Autodesk Inventor part; units mm, degrees
ref_plane "YZ Plane" through (0, 0, 0) normal (1, 0, 0) x (0, 1, 0)
ref_plane "XZ Plane" through (0, 0, 0) normal (0, 1, 0) x (-1, 0, 0)
ref_plane "XY Plane" through (0, 0, 0) normal (0, 0, 1) x (1, 0, 0)
sketch "Sketch1" plane through (0, 0, 0) normal (0, 0, 1) x (1, 0, 0)
  line L0 (5.5, 2.5) -> (5.5, 8)
  line L1 (5.5, 8) -> (3.5, 8)
  line L2 (3.5, 8) -> (3.5, 6.07)
  line L3 (3.5, 6.07) -> (0, 6.07)
  line L4 (5.5, 2.5) -> (0, 2.5)
  line L5 (0, 2.5) -> (0, 6.07)
  line L6 (-2.3, 0) -> (6.8, 0)
  line L7 (0, 0) -> (0, 17.5)
  line L8 (0, 9) -> (0, 2.5)
  line L9 (0, 15) -> (0, 9)
  point P0 (0, 4.285)
  point P1 (-1, 12)
  point P2 (4.5, 8)
  dimension "d0" = 5.5
  dimension "d1" = 3.5
  dimension "d2" = 6.07
  dimension "d3" = 8
  dimension "d4" = 2.5
  dimension "d8" = 1
revolve "Revolution1" add sketch "Sketch1" angle 360 about axis through (-10, 0, 0) along (1, 0, 0)
mirror "Mirror2" about plane through (0, 0, 0) normal (1, 0, 0) of "Revolution1"
properties part number "Idler_Pulley" material "Aluminum 6061"
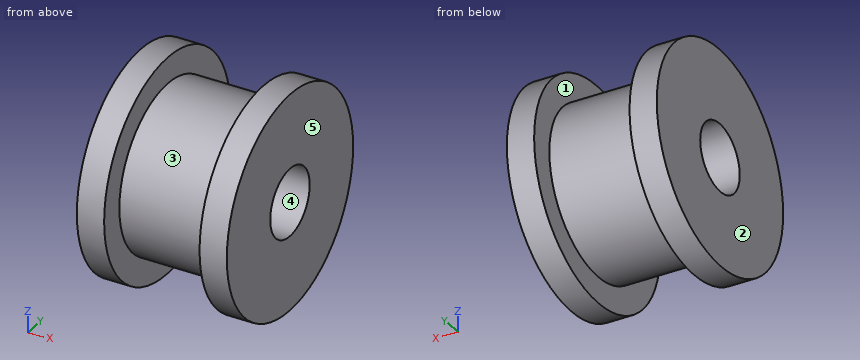
Can you work these out from the model? Positions are in its coordinate system, mm. Face numbers are marked on the shaded views. A direction names the side the tool comes from. Round coordinates to 2 decimals unless told otherwise and drop trailing zeros. Loops run counter-clockwise (first coordinate to the right, second up) from the corner with the lowest first, then second, coordinate; pieces in that order, holes last. Notation, with made-up numbers: (10.5, 49) -> (51.5, 49) arc R18 cw to (51.5, 83) -> close; hole circle Ø10 at (43, -12.75). An arc over 180 degrees is marked (long way). One line per item, written item: value. Start each with the question number.
1. For the marked faces 1 and 2, which set-ups out of +Z, -Z, +X, -X, +Y, -Y let a thin tool reach every point of the face, with its end or its side?
2. If we section it at A-A, the plane z = 0: Write out the boundary of the cut face in (x, y), then the cut area to 3 significant figures.
3. If we mould it in two halves opening along X, with no side actions, what happens to the marked faces 3, 4 and 5? For each: pulls with the +X half, pulls with the -X half, needs draft (parallel to the pull), parting line crosses it, or undercut.
4. If we section it at C-C, the plane x = -1: Write out the boundary of the cut face in (y, z).
5. If I drill on probe 1 along Z at (x, y) = (2.5, 0); probe 2 along X at (y, z) = (-5.75, -3.25); probe 3 along Y at (x, z) = (-3, -2.25), over which ranges is the centre line in solid material (lowest first)?
6. For pin 1 (1.5 mm diameter, centred on x = 2, y = 3.5, fed in from +Z); pin 2 (5 mm diameter, centred on x = -3.5, y = -5, fed in from +Z); pin 3 (2 mm diameter, centred on x = 0, y = -6.5, fed in from -Z); pin 4 (4 mm diameter, centred on y = 0, z = 0, fed in from +X), each with a flat end and sliding along its axis, tell me the tip position at first contact or that it passes through.
7. If we section it at D-D, the plane z = -5: Write out the boundary of the cut face in (x, y) (3 decimals).
Calculated:
1. face 1: none
1. face 2: +Z, -Z, -X, +Y, -Y
2. outline: (-5.5, -8) -> (-3.5, -8) -> (-3.5, -6.07) -> (3.5, -6.07) -> (3.5, -8) -> (5.5, -8) -> (5.5, -2.5) -> (-5.5, -2.5) -> close; (-5.5, 2.5) -> (5.5, 2.5) -> (5.5, 8) -> (3.5, 8) -> (3.5, 6.07) -> (-3.5, 6.07) -> (-3.5, 8) -> (-5.5, 8) -> close
2. area: 94.0 mm²
3. face 3: undercut
3. face 4: needs draft
3. face 5: pulls with the +X half
4. outline: circle Ø12.14 at (0, 0); hole circle Ø5 at (0, 0)
5. probe 1: z = -6.07 to -2.5, 2.5 to 6.07
5. probe 2: x = -5.5 to -3.5, 3.5 to 5.5
5. probe 3: y = -5.64 to -1.09, 1.09 to 5.64
6. pin 1: stops at z = 5.41
6. pin 2: stops at z = 7.6
6. pin 3: stops at z = -2.57
6. pin 4: passes through
7. outline: (-5.5, -6.245) -> (-3.5, -6.245) -> (-3.5, -3.442) -> (3.5, -3.442) -> (3.5, -6.245) -> (5.5, -6.245) -> (5.5, 6.245) -> (3.5, 6.245) -> (3.5, 3.442) -> (-3.5, 3.442) -> (-3.5, 6.245) -> (-5.5, 6.245) -> close
